Part print with two shaded views. Sizes in mm from the minimum x, y, z corner. A direction names the side the tool comes from. Coordinates: 2 decimals unless noted, no trailing zeros. Write each loop counter-clockwise with the first axis right and the second up, starting at its lowest first coordinate (ties: lowest second). Pieces come first, ordered by that corner, then holes.
Q1. Band-saw the part on D-D, the plane x = 24.5. Write the cut outline in (y, z).
Q2. Pin check, flat tips, straight feed: P1, Ø1, axis at x = 79.5, y = 42, coming from the -Z side; P2, Ø1.5, axis at x = 50, z = 10, coming from the -Y side; P3, Ø14, axis at x = 50.5, z = 11, coming from the +Y side; P4, Ø12, axis at y = 50.5, z = 26.5, coming from the +X side. Stop position of each tip, or through.
Q3. Which spindle directions (+Z, -Z, +X, -X, +Y, -Y) get a long thin tool onto all of the face, cutting with end or side? Do the marked faces 4, 5 and 6. Say none if no direction does.
Q4. Band-saw the part on A-A, the plane x = 11. Write the cut outline in (y, z), plus the area to 3 significant figures.
Q5. Band-saw the part on C-C, the plane x = 63.5. Write the cut outline in (y, z).
Q6. Drill centre lines: probe 1 along Z at (x, y) = (63.5, 27.5); probe 2 along Y at (x, z) = (63, 21.5); probe 3 along X at (y, z) = (3.5, 9.5). Where is each one in solid material? Low to high.
Q7. Pull direction Y, two halves, no side cores. Call the marked faces 1, 2 and 3: released by +Y, released by -Y, zero draft, split by the parting line, or undercut.
Q8. Band-saw the part on B-B, the plane z = 24. Write the cut outline in (x, y) (1 decimal), plus the area to 4 significant figures.
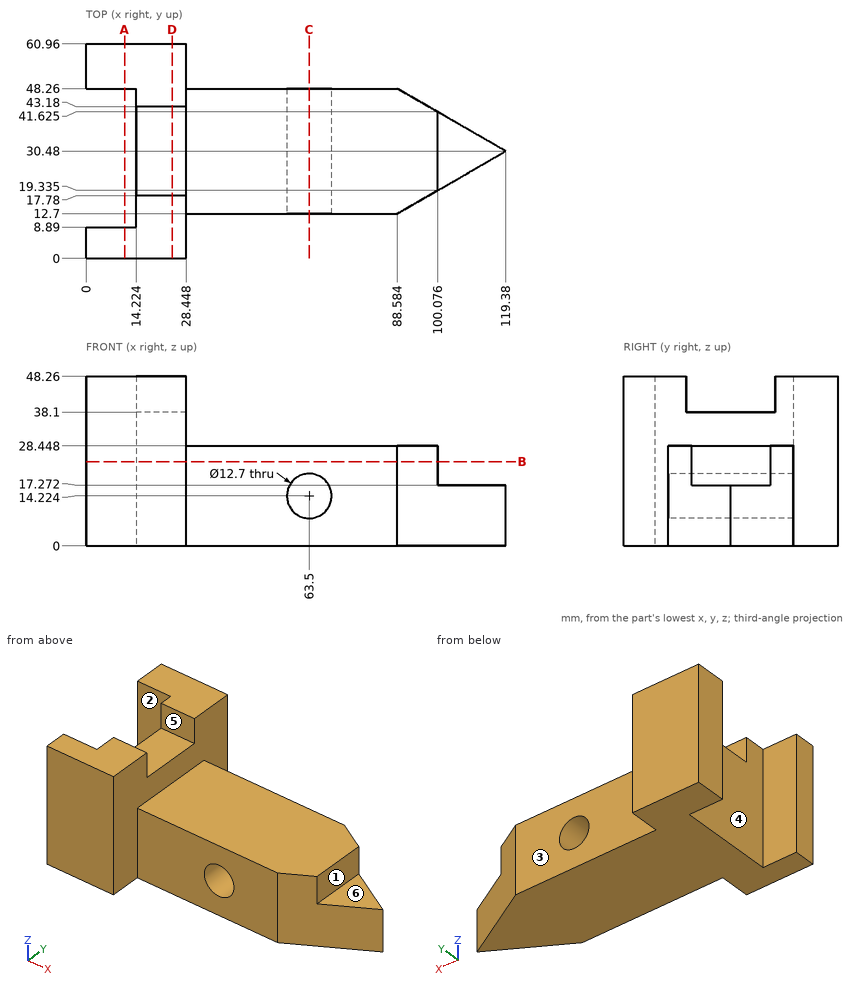
Answer sheet:
1. outline: (0, 0) - (60.96, 0) - (60.96, 48.26) - (43.18, 48.26) - (43.18, 38.1) - (17.78, 38.1) - (17.78, 48.26) - (0, 48.26) - close
2. P1: stops at z = 0
2. P2: stops at y = 12.7
2. P3: stops at y = 48.26
2. P4: stops at x = 95.1
3. face 4: +Z, -Z, -X
3. face 5: +Z, +X, -X
3. face 6: +Z, +X, +Y, -Y
4. outline: (0, 0) - (8.89, 0) - (8.89, 48.26) - (0, 48.26) - close; (48.26, 0) - (60.96, 0) - (60.96, 48.26) - (48.26, 48.26) - close
4. area: 1,040 mm2
5. outline: (12.7, 0) - (48.26, 0) - (48.26, 7.87) - (12.7, 7.87) - close; (12.7, 20.57) - (48.26, 20.57) - (48.26, 28.45) - (12.7, 28.45) - close
6. probe 1: z = 0 to 7.87, 20.57 to 28.45
6. probe 2: y = 12.7 to 48.26
6. probe 3: x = 0 to 28.45
7. face 1: zero draft
7. face 2: undercut
7. face 3: released by +Y
8. outline: (0, 0) - (28.4, 0) - (28.4, 12.7) - (88.6, 12.7) - (100.1, 19.3) - (100.1, 41.6) - (88.6, 48.3) - (28.4, 48.3) - (28.4, 61) - (0, 61) - (0, 48.3) - (14.2, 48.3) - (14.2, 8.9) - (0, 8.9) - close
8. area: 3,645 mm2
